CAD build for the part. Positions are in the model's coordinates, mm. A direction names the side the tool comes from. Give positions to 0.01 mm unless a question says otherwise; leave off trailing zeros. Order: outer loops, then holes, each group sorted by start corner. A loop starts at its lowest first (then second) coordinate and runs counter-clockwise, first axis right, second up. Notation, with made-up numbers: M 12,59.25 L 22,59.25 A30 cw 22,98.25 Z; hole C 74,5.5 d6. An arc over 180 degrees is marked long. Put each result on its own line as item: value. Start each with the question number.
1) Two-plate mould, pull along X, no slides. Class faces 4 (the face through (44.666, -25.144, 0.789)), 5 (the face through (-42.26, 0, 3)), 6 (the face through (48.1, 27.14, 0.79)): released by +X, released by -X, zero draft, split by the parting line, or undercut.
2) Drill centre lines: line 1 (X direction, y = -21.5, z = 2.5); line 2 (Y direction, x = 37, z = 3.2). Where is each one in solid material? Low to high. Write a range as [from, to].
3) Pin check, flat tips, straight feed: pin 1 (1.9 mm diameter, centred on x = 18.5, z = 3, fed in from -Y); pin 2 (0.7 mm diameter, centred on y = -6, z = 3, fed in from -X); pin 3 (1.8 mm diameter, centred on x = 46.165, y = 25.21, fed in from -Z); pin 4 (4 mm diameter, centred on x = -46.165, y = -25.21, fed in from +Z). Stop position of each tip, or through.
4) Tool access for faces 1 (the face through (-1, 27, 3)), 2 (the face through (42.26, 0, 3)), 3 (the face through (-1, -27, 3)): list every direction of +Z, -Z, +X, -X, +Y, -Y with a clear straight run to the whole face (end or side of a thin tool).
5) Cut at A-A (y = -17.5). Write the cut outline in (x, z).
6) Cut at B-B (x = 2.5). Write the cut outline in (y, z).
```python
from build123d import *

# Parameters (mm, degrees)
ESBO_O1_R                = 1.5
RESSALTO_EXTRUS_O1_DEPTH = 1.6
ESBO_O1_3_W              = 84.52
ESBO_O1_3_H              = 54
RESSALTO_EXTRUS_O2_DEPTH = 4


with BuildPart() as part:
    # Esbo_o1 → Ressalto-extrus_o1 (new body)
    with BuildSketch(Plane.XY):
        with BuildLine():
            Line((-46, 28), (46, 28))
            ThreePointArc((46, 28), (48.121320344, 27.121320344), (49, 25))
            Line((49, 25), (49, -25))
            ThreePointArc((49, -25), (48.121320344, -27.121320344), (46, -28))
            Line((46, -28), (-46, -28))
            ThreePointArc((-46, -28), (-48.121320344, -27.121320344), (-49, -25))
            Line((-49, -25), (-49, 25))
            ThreePointArc((-49, 25), (-48.121320344, 27.121320344), (-46, 28))
        make_face()
        with Locations((-46.165, 25.21)):
            Circle(ESBO_O1_R, mode=Mode.SUBTRACT)
        with Locations((46.165, 25.21)):
            Circle(ESBO_O1_R, mode=Mode.SUBTRACT)
        with Locations((-46.165, -25.21)):
            Circle(ESBO_O1_R, mode=Mode.SUBTRACT)
        with Locations((46.165, -25.21)):
            Circle(ESBO_O1_R, mode=Mode.SUBTRACT)
    extrude(amount=RESSALTO_EXTRUS_O1_DEPTH)

    # Esbo_o1_3 → Ressalto-extrus_o2 (add)
    with BuildSketch(Plane.XY):
        Rectangle(ESBO_O1_3_W, ESBO_O1_3_H)
    extrude(amount=RESSALTO_EXTRUS_O2_DEPTH)


solid = part.part
```
Solution:
1. face 4: undercut
1. face 5: released by -X
1. face 6: released by +X
2. line 1: [-42.26, 42.26]
2. line 2: [-27, 27]
3. pin 1: y = -27
3. pin 2: x = -42.26
3. pin 3: through
3. pin 4: z = 1.6
4. face 1: +Z, +X, -X, +Y
4. face 2: +Z, +X, +Y, -Y
4. face 3: +Z, +X, -X, -Y
5. outline: M -49,0 L 49,0 L 49,1.6 L 42.26,1.6 L 42.26,4 L -42.26,4 L -42.26,1.6 L -49,1.6 Z
6. outline: M -28,0 L 28,0 L 28,1.6 L 27,1.6 L 27,4 L -27,4 L -27,1.6 L -28,1.6 Z
